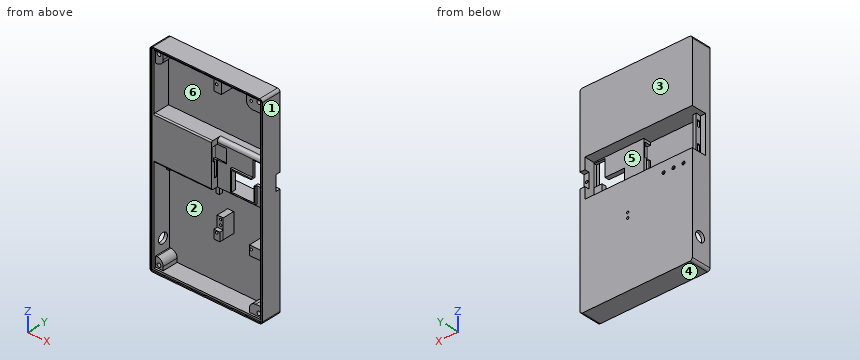
```python
from build123d import *

# Parameters (mm, degrees)
SKETCH1_W            = 90
SKETCH1_H            = 160
BOSS_EXTRUDE1_DEPTH  = 15
SKETCH2_W            = 46
SKETCH2_H            = 30
CUT_EXTRUDE1_DEPTH   = 12
SKETCH3_W            = 44
SKETCH3_H            = 30
CUT_EXTRUDE2_DEPTH   = 8
SHELL1_START         = -47.6
SHELL1_OUTLINE_W     = 85.2
SHELL1_OUTLINE_H     = 13
SHELL1_DEPTH         = 45.2
SHELL1_START_2       = -157.6
SHELL1_2_OUTLINE_W   = 85.2
SHELL1_2_OUTLINE_H   = 5
SHELL1_2_DEPTH       = 75.2
SKETCH7_W            = 39
SKETCH7_H            = 34.8
CUT_EXTRUDE6_DEPTH   = 5
SKETCH11_W           = 42.056152249
SKETCH11_H           = 30
CUT_EXTRUDE9_DEPTH   = 2
CUT_EXTRUDE7_DEPTH   = 10
CUT_EXTRUDE10_DEPTH  = 3
SKETCH14_W           = 90
SKETCH14_H           = 160
SKETCH14_W_2         = 88.2
SKETCH14_H_2         = 158.2
BOSS_EXTRUDE2_DEPTH  = 1
SKETCH22_W           = 4
SKETCH22_H           = 30
BOSS_EXTRUDE6_DEPTH  = 8
SKETCH26_W           = 4
SKETCH26_H           = 12
CUT_EXTRUDE20_DEPTH  = 3.8
SKETCH27_R           = 1
CUT_EXTRUDE21_DEPTH  = 3
BOSS_EXTRUDE9_DEPTH  = 1.5
SKETCH40_R           = 4
CUT_EXTRUDE24_DEPTH  = 5
FILLET1_R            = 3
SKETCH44_W           = 85.2
SKETCH44_H           = 75.2
CUT_EXTRUDE25_DEPTH  = 9
SKETCH46_W           = 4.8
SKETCH46_H           = 15.6
BOSS_EXTRUDE15_DEPTH = 12.5
SKETCH6_R            = 0.9
CUT_EXTRUDE26_DEPTH  = 29.4
SKETCH47_W           = 33.8
SKETCH47_H           = 48
SKETCH47_W_2         = 6
SKETCH47_H_2         = 8
BOSS_EXTRUDE16_DEPTH = 12.5
SKETCH49_W           = 38.660197992
SKETCH49_H           = 10
SKETCH49_W_2         = 6
BOSS_EXTRUDE17_DEPTH = 11.5
CUT_EXTRUDE28_REACH  = 186.071
SKETCH50_W           = 22
SKETCH50_H           = 7
SKETCH50_W_2         = 20
SKETCH50_H_2         = 9
FILLET4_R            = 2
SKETCH51_R           = 1.5
CUT_EXTRUDE29_DEPTH  = 6
CUT_EXTRUDE30_DEPTH  = 3
SKETCH52_R           = 1
CUT_EXTRUDE31_DEPTH  = 3
SKETCH54_W           = 2.470433815
SKETCH54_H           = 30
BOSS_EXTRUDE18_DEPTH = 6
SKETCH55_W           = 5
SKETCH55_H           = 2
CUT_EXTRUDE32_DEPTH  = 3
FILLET5_R            = 1
SKETCH56_R           = 1.25
CUT_EXTRUDE33_DEPTH  = 3
SKETCH57_W           = 2.5
SKETCH57_H           = 8
BOSS_EXTRUDE19_DEPTH = 3
CUT_EXTRUDE36_REACH  = 186.071
SKETCH59_W           = 10.104623882
SKETCH59_H           = 32.567789254
SKETCH60_W           = 23.695376118
SKETCH60_H           = 48.017621291
CUT_EXTRUDE37_DEPTH  = 9.5
FILLET3_R            = 5


# Read off the part's stored shape, not the designer's step: Shell1
with BuildPart() as part:
    # Sketch1 → Boss-Extrude1 (new body)
    with BuildSketch(Plane(origin=(0, 0, 0), x_dir=(1, 0, 0), z_dir=(0, 1, 0))):
        with Locations((45, 80)):
            Rectangle(SKETCH1_W, SKETCH1_H)
    extrude(amount=BOSS_EXTRUDE1_DEPTH)

    # Sketch2 → Cut-Extrude1 (cut)
    with BuildSketch(Plane(origin=(0, 15, 0), x_dir=(1, 0, 0), z_dir=(0, 1, 0))):
        with Locations((23, 65)):
            Rectangle(SKETCH2_W, SKETCH2_H)
    extrude(amount=-CUT_EXTRUDE1_DEPTH, mode=Mode.SUBTRACT)

    # Sketch3 → Cut-Extrude2 (cut)
    with BuildSketch(Plane(origin=(0, 15, 0), x_dir=(1, 0, 0), z_dir=(0, 1, 0))):
        with Locations((68, 65)):
            Rectangle(SKETCH3_W, SKETCH3_H)
    extrude(amount=-CUT_EXTRUDE2_DEPTH, mode=Mode.SUBTRACT)

    # Shell1 outline → Shell1 (cut)
    with BuildSketch(Plane.XY.offset(SHELL1_START)):
        with Locations((45, 6.5)):
            Rectangle(SHELL1_OUTLINE_W, SHELL1_OUTLINE_H)
    extrude(amount=SHELL1_DEPTH, mode=Mode.SUBTRACT)

    # Shell1 2 outline → Shell1 2 (cut)
    with BuildSketch(Plane.XY.offset(SHELL1_START_2)):
        with Locations((45, 2.5)):
            Rectangle(SHELL1_2_OUTLINE_W, SHELL1_2_OUTLINE_H)
    extrude(amount=SHELL1_2_DEPTH, mode=Mode.SUBTRACT)

    # Sketch7 → Cut-Extrude6 (cut)
    with BuildSketch(Plane.XZ):
        with Locations((68.1, -65)):
            Rectangle(SKETCH7_W, SKETCH7_H)
    extrude(amount=-CUT_EXTRUDE6_DEPTH, mode=Mode.SUBTRACT)

    # Sketch11 → Cut-Extrude9 (cut)
    with BuildSketch(Plane(origin=(0, 3, 0), x_dir=(1, 0, 0), z_dir=(0, 1, 0))):
        with Locations((24.971923875, 65)):
            Rectangle(SKETCH11_W, SKETCH11_H)
    extrude(amount=-CUT_EXTRUDE9_DEPTH, mode=Mode.SUBTRACT)

    # Sketch8 → Cut-Extrude7 (cut)
    with BuildSketch(Plane.ZY.offset(-46)):
        Polygon((-63, 1), (-63, 2.5), (-75, 2.5), (-75, 4.5), (-63, 4.5), (-63, 6), (-52, 6), (-52, 4.5), (-52, 1), align=None)
    extrude(amount=-CUT_EXTRUDE7_DEPTH, mode=Mode.SUBTRACT)

    # Sketch12 → Cut-Extrude10 (cut)
    with BuildSketch(Plane(origin=(0, 7, 0), x_dir=(1, 0, 0), z_dir=(0, 1, 0))):
        Polygon((79.361885724, 68), (79.361885724, 80), (61.361885724, 80), (61.361885724, 64.5), (77.04695331, 64.5), (77.04695331, 51), (85.714801791, 51), (85.714801791, 68), align=None)
    extrude(amount=-CUT_EXTRUDE10_DEPTH, mode=Mode.SUBTRACT)

    # Sketch14 → Boss-Extrude2 (add)
    with BuildSketch(Plane.XZ):
        with Locations((45, -80)):
            Rectangle(SKETCH14_W, SKETCH14_H)
        with Locations((45, -80)):
            Rectangle(SKETCH14_W_2, SKETCH14_H_2, mode=Mode.SUBTRACT)
    extrude(amount=BOSS_EXTRUDE2_DEPTH)

    # Sketch22 → Boss-Extrude6 (add)
    with BuildSketch(Plane(origin=(0, 7, 0), x_dir=(1, 0, 0), z_dir=(0, 1, 0))):
        with Locations((88, 65)):
            Rectangle(SKETCH22_W, SKETCH22_H)
    extrude(amount=BOSS_EXTRUDE6_DEPTH)

    # Sketch26 → Cut-Extrude20 (cut)
    with BuildSketch(Plane(origin=(0, 15, 0), x_dir=(1, 0, 0), z_dir=(0, 1, 0))):
        with Locations((88, 65)):
            Rectangle(SKETCH26_W, SKETCH26_H)
    extrude(amount=-CUT_EXTRUDE20_DEPTH, mode=Mode.SUBTRACT)

    # Sketch27 → Cut-Extrude21 (cut)
    with BuildSketch(Plane(origin=(0, 11.2, 0), x_dir=(1, 0, 0), z_dir=(0, 1, 0))):
        with Locations(Location((88, 65, 0), (0, 0, 270))):
            Circle(SKETCH27_R)
    extrude(amount=-CUT_EXTRUDE21_DEPTH, mode=Mode.SUBTRACT)

    # Sketch36 → Boss-Extrude9 (add)
    with BuildSketch(Plane.XZ.offset(-5)):
        Polygon((77.04695331, -63.5), (60.361885724, -63.5), (60.361885724, -81), (80.361885724, -81), (80.361885724, -68), (79.361885724, -68), (79.361885724, -80), (61.361885724, -80), (61.361885724, -64.5), (77.04695331, -64.5), align=None)
    extrude(amount=BOSS_EXTRUDE9_DEPTH)

    # Sketch40 → Cut-Extrude24 (cut)
    with BuildSketch(Plane.ZY):
        with Locations((-140, 8)):
            Circle(SKETCH40_R)
    extrude(amount=-CUT_EXTRUDE24_DEPTH, mode=Mode.SUBTRACT)

    # Fillet1
    fillet1_edges = [part.edges().sort_by_distance(p)[0] for p in [
        (68.1, 5, -47.6),
    ]]
    fillet(fillet1_edges, radius=FILLET1_R)

    # Sketch44 → Cut-Extrude25 (cut)
    with BuildSketch(Plane.XZ.offset(-5)):
        with Locations((45, -120)):
            Rectangle(SKETCH44_W, SKETCH44_H)
    extrude(amount=-CUT_EXTRUDE25_DEPTH, mode=Mode.SUBTRACT)

    # Sketch46 → Boss-Extrude15 (add)
    with BuildSketch(Plane.XZ.offset(-14)):
        with Locations((51.4, -109.8)):
            Rectangle(SKETCH46_W, SKETCH46_H)
    extrude(amount=BOSS_EXTRUDE15_DEPTH)

    # Sketch6 → Cut-Extrude26 (cut)
    with BuildSketch(Plane(origin=(0, 15, 0), x_dir=(1, 0, 0), z_dir=(0, 1, 0))):
        with Locations(Location((51.75, 108, 0), (0, 0, 270))):
            Circle(SKETCH6_R)
        with Locations(Location((51.75, 104, 0), (0, 0, 270))):
            Circle(SKETCH6_R)
    extrude(amount=-CUT_EXTRUDE26_DEPTH, mode=Mode.SUBTRACT)

    # Sketch47 → Boss-Extrude16 (add)
    with BuildSketch(Plane.XZ.offset(-14)):
        with Locations((70.7, -133.6)):
            Rectangle(SKETCH47_W, SKETCH47_H)
        with Locations((5.4, -153.6)):
            Rectangle(SKETCH47_W_2, SKETCH47_H_2)
    extrude(amount=BOSS_EXTRUDE16_DEPTH)

    # Sketch49 → Boss-Extrude17 (add)
    with BuildSketch(Plane.XZ.offset(-13)):
        with Locations((68.269901004, -7.4)):
            Rectangle(SKETCH49_W, SKETCH49_H)
        with Locations((5.4, -7.4)):
            Rectangle(SKETCH49_W_2, SKETCH49_H)
    extrude(amount=BOSS_EXTRUDE17_DEPTH)

    # Cut-Extrude28: up to this face of the body (flat: up to its plane)
    cut_extrude28_end = Plane(part.part.faces().sort_by_distance((36.360749588, 14, -115.08476112))[0])
    # Sketch50 → Cut-Extrude28 (cut, up to the picked face)
    with BuildSketch(Plane.XZ.offset(-1.5), mode=Mode.PRIVATE) as cut_extrude28_sk1:
        with Locations((64.8, -113.1)):
            Rectangle(SKETCH50_W, SKETCH50_H)
    cut_extrude28_tool1 = split(extrude(cut_extrude28_sk1.sketch, amount=-CUT_EXTRUDE28_REACH, mode=Mode.PRIVATE), bisect_by=cut_extrude28_end, keep=Keep.BOTH, mode=Mode.PRIVATE)
    # Sketch50 → Cut-Extrude28 (cut, up to the picked face)
    with BuildSketch(Plane.XZ.offset(-1.5), mode=Mode.PRIVATE) as cut_extrude28_sk2:
        with Locations((64.939802008, -7.9)):
            Rectangle(SKETCH50_W_2, SKETCH50_H_2)
    cut_extrude28_tool2 = split(extrude(cut_extrude28_sk2.sketch, amount=-CUT_EXTRUDE28_REACH, mode=Mode.PRIVATE), bisect_by=cut_extrude28_end, keep=Keep.BOTH, mode=Mode.PRIVATE)
    add(cut_extrude28_tool1.solids().sort_by(Axis((64.8, 1.5, -113.1), (0, 1, 0)))[0], mode=Mode.SUBTRACT)
    add(cut_extrude28_tool2.solids().sort_by(Axis((64.939802, 1.5, -7.9), (0, 1, 0)))[0], mode=Mode.SUBTRACT)

    # Fillet4
    fillet4_edges = [part.edges().sort_by_distance(p)[0] for p in [
        (0, 7, -160),
        (90, 7, -160),
        (90, 7, 0),
        (0, 7, 0),
    ]]
    fillet(fillet4_edges, radius=FILLET4_R)

    # Sketch51 → Cut-Extrude29 (cut)
    with BuildSketch(Plane.XZ.offset(-1.5)):
        with Locations(Location((85, -155, 0), (0, 0, 270))):
            Circle(SKETCH51_R)
        with Locations(Location((85, -5, 0), (0, 0, 270))):
            Circle(SKETCH51_R)
        with Locations(Location((5, -5, 0), (0, 0, 270))):
            Circle(SKETCH51_R)
        with Locations(Location((5, -155, 0), (0, 0, 270))):
            Circle(SKETCH51_R)
    extrude(amount=-CUT_EXTRUDE29_DEPTH, mode=Mode.SUBTRACT)

    # Sketch53 → Cut-Extrude30 (cut)
    with BuildSketch(Plane.XZ.offset(-1.5)):
        Polygon((75.8, -109.6), (77.495376118, -109.6), (77.495376118, -157.6), (53.787002796, -157.6), (53.787002796, -110.656453849), (49, -110.656453849), (49, -102), (53.8, -102), (53.8, -116.6), (75.8, -116.6), align=None)
    extrude(amount=-CUT_EXTRUDE30_DEPTH, mode=Mode.SUBTRACT)

    # Sketch52 → Cut-Extrude31 (cut)
    with BuildSketch(Plane.XZ.offset(-1.5)):
        with Locations(Location((78.9, -6.622682824, 0), (0, 0, 270))):
            Circle(SKETCH52_R)
        with Locations(Location((51.19, -6.622682824, 0), (0, 0, 270))):
            Circle(SKETCH52_R)
        with Locations(Location((78.9, -112.202682824, 0), (0, 0, 270))):
            Circle(SKETCH52_R)
        with Locations(Location((51.19, -112.202682824, 0), (0, 0, 270))):
            Circle(SKETCH52_R)
    extrude(amount=-CUT_EXTRUDE31_DEPTH, mode=Mode.SUBTRACT)

    # Sketch54 → Boss-Extrude18 (add)
    with BuildSketch(Plane(origin=(0, 1, 0), x_dir=(1, 0, 0), z_dir=(0, 1, 0))):
        with Locations((5.179064659, 65)):
            Rectangle(SKETCH54_W, SKETCH54_H)
    extrude(amount=BOSS_EXTRUDE18_DEPTH)

    # Sketch55 → Cut-Extrude32 (cut)
    with BuildSketch(Plane.ZY.offset(-3.943847751)):
        with Locations((-73.5, 5)):
            Rectangle(SKETCH55_W, SKETCH55_H)
        with Locations((-56.5, 5)):
            Rectangle(SKETCH55_W, SKETCH55_H)
    extrude(amount=-CUT_EXTRUDE32_DEPTH, mode=Mode.SUBTRACT)

    # Fillet5
    fillet5_edges = [part.edges().sort_by_distance(p)[0] for p in [
        (25.5, 0, -82.4),
        (25.5, 0, -47.6),
    ]]
    fillet(fillet5_edges, radius=FILLET5_R)

    # Sketch56 → Cut-Extrude33 (cut)
    with BuildSketch(Plane(origin=(0, 15, 0), x_dir=(1, 0, 0), z_dir=(0, 1, 0))):
        with Locations(Location((7, 88, 0), (0, 0, 270))):
            Circle(SKETCH56_R)
        with Locations(Location((15, 88, 0), (0, 0, 270))):
            Circle(SKETCH56_R)
        with Locations(Location((23, 88, 0), (0, 0, 270))):
            Circle(SKETCH56_R)
    extrude(amount=-CUT_EXTRUDE33_DEPTH, mode=Mode.SUBTRACT)

    # Sketch57 → Boss-Extrude19 (add)
    with BuildSketch(Plane.XZ.offset(-14)):
        with Locations((3.65, -88.4)):
            Rectangle(SKETCH57_W, SKETCH57_H)
        with Locations((43.65, -88.4)):
            Rectangle(SKETCH57_W, SKETCH57_H)
    extrude(amount=BOSS_EXTRUDE19_DEPTH)

    # Cut-Extrude36: up to this face of the body (flat: up to its plane)
    cut_extrude36_end = Plane(part.part.faces().sort_by_distance((37.453503344, 14, -115.328530292))[0])
    # Sketch59 → Cut-Extrude36 (cut, up to the picked face)
    with BuildSketch(Plane.XZ.offset(-1.5), mode=Mode.PRIVATE) as cut_extrude36_sk1:
        with Locations((82.547688059, -133.39637261)):
            Rectangle(SKETCH59_W, SKETCH59_H)
    cut_extrude36_tool1 = split(extrude(cut_extrude36_sk1.sketch, amount=-CUT_EXTRUDE36_REACH, mode=Mode.PRIVATE), bisect_by=cut_extrude36_end, keep=Keep.BOTH, mode=Mode.PRIVATE)
    add(cut_extrude36_tool1.solids().sort_by(Axis((82.547688, 1.5, -133.396373), (0, 1, 0)))[0], mode=Mode.SUBTRACT)

    # Sketch60 → Cut-Extrude37 (cut)
    with BuildSketch(Plane.XZ.offset(-4.5)):
        with Locations((65.647688059, -133.591189355)):
            Rectangle(SKETCH60_W, SKETCH60_H)
    extrude(amount=-CUT_EXTRUDE37_DEPTH, mode=Mode.SUBTRACT)

    # Fillet3
    fillet3_edges = [part.edges().sort_by_distance(p)[0] for p in [
        (8.4, 7.75, -149.6),
        (8.4, 7.25, -12.4),
        (74.939802008, 7.25, -12.4),
        (77.495376118, 7.75, -149.680267237),
    ]]
    fillet(fillet3_edges, radius=FILLET3_R)


solid = part.part
```
Geometry: final body of the model. Coordinates: model frame, mm. Face numbers are marked on the shaded views. A direction names the side the tool comes from. Round coordinates to 2 decimals unless told otherwise and drop trailing zeros. Order: outer loops, then holes, each group sorted by start corner. A loop starts at its lowest first (then second) coordinate and runs counter-clockwise, first axis right, second up. Notation, with made-up numbers: (63.25, 0) -> (108.25, 0) arc R25 cw to (108.25, 31) -> close; hole circle Ø8 at (39, 12.25). An arc over 180 degrees is marked (long way). Use CSV: the item, a comma, the result in double quotes. Start each with the question number.
1) Section B-B (z = -45). Return the cut outline in (x, y).
2) Draft query along X for the marked faces 1, 2 and 3. Return one class per face: +X half, -X half, draft (parallel to the pull), parting line (faces both ways), or undercut.
3) Material intervals for line 1 along X through (y, z) = (7.25, -112.5); line 2 along Z through (x, y) = (42, 4.5); line 3 along X through (y, z) = (14.45, -88), sorted ascending. Write a range as from..to.
4) First-contact query: pin 1 Ø7 at (x, z) = (68, -7) entering from -Y; pin 2 Ø1.2 at (x, z) = (5, -57.5) entering from +Y; pin 3 Ø3 at (x, z) = (2, -61.5) entering from +Y; pin 4 Ø5 at (x, z) = (76.5, -67.5) entering from +Y. Flat tips, straight axial feed; report the tip coordinate or a pass-through.
5) Section A-A (z = -140). Return the cut outline in (x, y).
6) Set-up query: the marked faces 4, 5 and 6. Return all of +Z, -Z, +X, -X, +Y, -Y with unobstructed straight access to the full face (end or side cutting, diameter ignored); none if empty.
Returned:
1,outline,"(0, -1) -> (0.9, -1) -> (0.9, 0) -> (2.4, 0) -> (2.4, 13) -> (87.6, 13) -> (87.6, 0) -> (89.1, 0) -> (89.1, -1) -> (90, -1) -> (90, 15) -> (0, 15) -> close"
2,face 1,"+X half"
2,face 2,"undercut"
2,face 3,"draft"
3,line 1,"x = 0..2.4, 49..53.8, 77.5..90"
3,line 2,"z = -160..-157.6, -82.4..-80, -50..-47.6, -2.4..0"
3,line 3,"x = 0..5.75, 8.25..13.75, 16.25..21.75, 24.25..90"
4,pin 1,"stops at y = 14"
4,pin 2,"stops at y = 7"
4,pin 3,"stops at y = 3"
4,pin 4,"passes through"
5,outline,"(0, -1) -> (0.9, -1) -> (0.9, 0) -> (2.4, 0) -> (2.4, 4) -> (0, 4) -> close; (0, 12) -> (2.4, 12) -> (2.4, 14) -> (87.6, 14) -> (87.6, 0) -> (89.1, 0) -> (89.1, -1) -> (90, -1) -> (90, 15) -> (0, 15) -> close"
6,face 4,"-Z, +X, -X, +Y, -Y"
6,face 5,"-X, +Y"
6,face 6,"-Y"
